Design review of the part built by this model. Coordinates are the model's own, in mm. A direction names the side the tool comes from. Coordinates: 2 decimals unless noted, no trailing zeros. Loops run counter-clockwise (first coordinate to the right, second up) from the corner with the lowest first, then second, coordinate; pieces in that order, holes last. Notation, with made-up numbers: M 59.25,32.25 L 89.25,32.25 A20 cw 89.25,64.25 Z; hole C 50,-7 d3. An arc over 180 degrees is marked long. Answer as a JSON object with one key per item and string values. Group by question number.
1. Draft analysis for pull direction Z (two halves, no side actions). For faces 1 (the cylindrical face through (54.797, 1.141, 5.07)), 2 (the cylindrical face through (5.01, 14.54, 47.47)), 3 (the flat face through (31, 25, 10)), 4 (the flat face through (4, 26.725, 44)), state which applies: +Z half, -Z half, draft (parallel to the pull), parting line (faces both ways), or undercut.
2. Consider section C-C (x = 12). State the section outline as (y, z) points.
3. Consider section A-A (y = 35). State the section outline as (x, z) points.
4. Consider section D-D (y = 42.5). State the section outline as (x, z) points.
5. Machinability: for faces 5 (the flat face through (3, 25, 58)), 6 (the flat face through (1, 27.76, 44)), 7 (the flat face through (4, 17, 44)), 8 (the flat face through (25.129, 47.972, 35.046)), 9 (the flat face through (17, 4, 28)), which of the approach directions +Z, -Z, +X, -X, +Y, -Y give a long, thin tool a straight path to every point of the face, cutting with its end or side? Answer none if there is none.
6. To check wall thickness, follow probe 1 along Z at (x, y) = (2, 15); probe 2 along Z at (x, y) = (5.55, 15); probe 3 along Y at (x, z) = (8.5, 51). State the ranges of each line that lie inside material, in increasing order.
7. Consider section B-B (z = 24). Count the separate pieces of the cut face and the enclosed holes in it, then the cut area to 3 significant figures.
8. Insertion check: pin 1 (4.5 mm diameter, centred on x = 3.5, y = 25.5, fed in from -Z); pin 2 (1.6 mm diameter, centred on x = 1, z = 27, fed in from -Y); pin 3 (7.5 mm diameter, centred on y = 35.5, z = 43.5, fed in from +X); pin 4 (3.5 mm diameter, centred on y = 15.5, z = 23, fed in from +X). Each pin has a flat end and moves straight along its axis. Give the tip position at first contact, or say it passes through.
from build123d import *

# Parameters (mm, degrees)
F0_W      = 56
F0_H      = 50
F1_DEPTH  = 10
F2_W      = 40
F2_H      = 4
F3_DEPTH  = 48
F5_DEPTH  = 50.001
F6_R      = 4
F7_W      = 1.035
F7_H      = 16
F8_DEPTH  = 2
F7_W_2    = 3.45
F9_DEPTH  = 6
F10_R     = 3.5
F10_R_2   = 1.5
F11_DEPTH = 2
F12_DEPTH = 6


with BuildPart() as f1:
    # F0 (on Top) → F1 (new body)
    with BuildSketch(Plane.XY):
        with Locations((28, 25)):
            Rectangle(F0_W, F0_H)
    extrude(amount=F1_DEPTH)

    # F2 (on face) → F3 (join)
    with BuildSketch(Plane.XY.offset(10)):
        Polygon((6, 50), (0, 50), (0, 0), (6, 0), (6, 4), (6, 46), align=None)
        with Locations((26, 48)):
            Rectangle(F2_W, F2_H)
        with Locations((26, 2)):
            Rectangle(F2_W, F2_H)
    extrude(amount=F3_DEPTH)

    # F4 (on face) → F5 (cut, through all)
    with BuildSketch(Plane.XZ):
        Polygon((6, 58), (46, 10), (46, 58), align=None)
    extrude(amount=-F5_DEPTH, mode=Mode.SUBTRACT)

    # F6
    f6_edges = [f1.edges().sort_by_distance(p)[0] for p in [
        (0, 0, 29),
        (56, 0, 5),
        (46, 2, 10),
        (46, 48, 10),
        (56, 50, 5),
        (0, 50, 29),
    ]]
    fillet(f6_edges, radius=F6_R)

    # F7 (on face) → F8 (cut)
    with BuildSketch(Plane(origin=(0, 0, 0), x_dir=(0, -1, 0), z_dir=(-1, 0, 0))):
        with Locations((-27.2425, 44)):
            Rectangle(F7_W, F7_H)
        with Locations((-22.7575, 44)):
            Rectangle(F7_W, F7_H)
        with Locations((-22.7575, 24)):
            Rectangle(F7_W, F7_H)
        with Locations((-27.2425, 24)):
            Rectangle(F7_W, F7_H)
    extrude(amount=-F8_DEPTH, mode=Mode.SUBTRACT)

    # F7 (on face) → F9 (cut, through all)
    with BuildSketch(Plane(origin=(0, 0, 0), x_dir=(0, -1, 0), z_dir=(-1, 0, 0))):
        with Locations((-25, 44)):
            Rectangle(F7_W_2, F7_H)
        with Locations((-25, 24)):
            Rectangle(F7_W_2, F7_H)
    extrude(amount=-F9_DEPTH, mode=Mode.SUBTRACT)

    # F10 (on face) → F11 (cut)
    with BuildSketch(Plane.YZ.offset(6)):
        with Locations((15, 44)):
            Circle(F10_R)
        with Locations((15, 44)):
            Circle(F10_R_2, mode=Mode.SUBTRACT)
        with Locations((35, 44)):
            Circle(F10_R)
        with Locations((35, 44)):
            Circle(F10_R_2, mode=Mode.SUBTRACT)
        with Locations((35, 24)):
            Circle(F10_R)
        with Locations((35, 24)):
            Circle(F10_R_2, mode=Mode.SUBTRACT)
        with Locations((15, 24)):
            Circle(F10_R)
        with Locations((15, 24)):
            Circle(F10_R_2, mode=Mode.SUBTRACT)
    extrude(amount=-F11_DEPTH, mode=Mode.SUBTRACT)

    # F10 (on face) → F12 (cut, through all)
    with BuildSketch(Plane.YZ.offset(6)):
        with Locations((15, 44)):
            Circle(F10_R_2)
        with Locations((35, 44)):
            Circle(F10_R_2)
        with Locations((35, 24)):
            Circle(F10_R_2)
        with Locations((15, 24)):
            Circle(F10_R_2)
    extrude(amount=-F12_DEPTH, mode=Mode.SUBTRACT)


solid = f1.part
Findings below:
{
 "1": {"face 1": "draft", "face 2": "undercut", "face 3": "+Z half", "face 4": "undercut"},
 "2": {"outline": "M 0,0 L 50,0 L 50,50.8 L 46,50.8 L 46,10 L 4,10 L 4,50.8 L 0,50.8 Z"},
 "3": {"outline": "M 0,0 L 56,0 L 56,10 L 6,10 L 6,20.5 L 4,20.5 L 4,22.5 L 0,22.5 Z; M 0,25.5 L 4,25.5 L 4,27.5 L 6,27.5 L 6,40.5 L 4,40.5 L 4,42.5 L 0,42.5 Z; M 0,45.5 L 4,45.5 L 4,47.5 L 6,47.5 L 6,58 L 0,58 Z"},
 "4": {"outline": "M 0,0 L 56,0 L 56,10 L 6,10 L 6,58 L 0,58 Z"},
 "5": {"face 5": "+Z, +X, -X, +Y, -Y", "face 6": "-X", "face 7": "+X", "face 8": "+Z, +X, +Y, -Y", "face 9": "+Z, +X"},
 "6": {"probe 1": "z = 0 to 22.5, 25.5 to 42.5, 45.5 to 58", "probe 2": "z = 0 to 20.5, 27.5 to 40.5, 47.5 to 58", "probe 3": "y = 0 to 4, 46 to 50"},
 "7": {"separate pieces": "4", "enclosed holes": "0", "area": "443 mm^2"},
 "8": {"pin 1": "stops at z = 0", "pin 2": "stops at y = 0.66", "pin 3": "stops at x = 6", "pin 4": "stops at x = 4"}
}
